The listing builds one solid part. Answer for the finished solid, in the listing's coordinates (mm). A direction names the side the tool comes from. Give positions to 0.01 mm unless a question says otherwise; leave off trailing zeros. Order: outer loops, then holes, each group sorted by start corner. A loop starts at its lowest first (then second) coordinate and runs counter-clockwise, first axis right, second up. Notation, with made-up numbers: (19.25, 87) - (63.25, 87) arc R15 cw to (63.25, 91) - close; hole circle Ø5 at (39.25, 38.5). An arc over 180 degrees is marked (long way). Answer as a JSON object with one key per item and string values. Group by question number.
Q1. Given pin 1 (3 mm diameter, centred on y = -23.5, z = 1.5, fed in from -X); pin 2 (5 mm diameter, centred on y = 24.5, z = -26, fed in from +X), each flat-ended and moving along its own axis, determine where each tip first touches the part or whether it passes through.
Q2. A cutting plane is placed at D-D, the plane z = -1. Give the vertices of the cut face in (x, y), and give its area (3 significant figures).
Q3. For faces 1 (the face through (0, 22, -26)), 2 (the face through (0, -29, 26)), 3 (the face through (6.35, 0, 1)), determine the directions among +Z, -Z, +X, -X, +Y, -Y from which every point of the face is accessible in a straight line to the end or side of a thin tool.
Q4. The mould has two halves that part along Z. Classify faces 4 (the face through (-3.219, -21.384, 27.96)), 5 (the face through (0, -31.75, 1)), 6 (the face through (0, 0, -38.1)): released by +Z, released by -Z, zero draft, split by the parting line, or undercut.
Q5. Consider line 1 (Y direction, x = 5.5, z = -22.5); line 2 (Y direction, x = -1.5, z = -2.5); line 3 (X direction, y = -26.5, z = 28.5). Determine where each line is inside the solid, lowest interval first.
Q6. A cutting plane is placed at A-A, the plane y = -25.4. Count the separate pieces of the cut face and the enclosed holes in it, and give its area (3 significant figures).
from build123d import *

# Parameters (mm, degrees)
BOSS_EXTRUDE1_DEPTH                           = 38.1
F_1_4_20_THREADED_C_BORE_D                    = 6.35
F_1_4_20_THREADED_C_BORE_CBORE_D              = 9.525
F_1_4_20_THREADED_C_BORE_CBORE_DEPTH          = 6.35
F_1_4_20_THREADED_C_BORE_OPPOSITE_D           = 6.35
F_1_4_20_THREADED_C_BORE_OPPOSITE_CBORE_D     = 9.525
F_1_4_20_THREADED_C_BORE_OPPOSITE_CBORE_DEPTH = 6.35


with BuildPart() as part:
    # Sketch2 → Boss-Extrude1 (new, symmetric)
    with BuildSketch(Plane.XY):
        Polygon((-6.35, 31.75), (6.35, 31.75), (6.35, -19.05), (6.35, -31.75), (-6.35, -31.75), (-6.35, 19.05), align=None)
    extrude(amount=BOSS_EXTRUDE1_DEPTH, both=True)

    # 1/4"-20 threaded c-bore (through all)
    with Locations(Plane.ZY.offset(6.35)):
        with Locations((-25.4, -25.4), (0, -25.4), (25.4, -25.4)):
            CounterBoreHole(F_1_4_20_THREADED_C_BORE_D / 2, F_1_4_20_THREADED_C_BORE_CBORE_D / 2, F_1_4_20_THREADED_C_BORE_CBORE_DEPTH)

    # 1/4"-20 threaded c-bore opposite (through all)
    with Locations(Plane(origin=(6.35, 0, 0), x_dir=(0, 0, -1), z_dir=(1, 0, 0))):
        with Locations((-25.4, 25.4), (0, 25.4), (25.4, 25.4)):
            CounterBoreHole(F_1_4_20_THREADED_C_BORE_OPPOSITE_D / 2, F_1_4_20_THREADED_C_BORE_OPPOSITE_CBORE_D / 2, F_1_4_20_THREADED_C_BORE_OPPOSITE_CBORE_DEPTH)


solid = part.part
Reply:
{
 "1": {"pin 1": "stops at x = 0", "pin 2": "stops at x = 0"},
 "2": {"outline": "(-6.35, -31.75) - (6.35, -31.75) - (6.35, -28.41) - (0, -28.41) - (0, -30.06) - (-6.35, -30.06) - close; (-6.35, -20.74) - (0, -20.74) - (0, -22.39) - (6.35, -22.39) - (6.35, 20.74) - (0, 20.74) - (0, 22.39) - (-6.35, 22.39) - close; (-6.35, 28.41) - (0, 28.41) - (0, 30.06) - (6.35, 30.06) - (6.35, 31.75) - (-6.35, 31.75) - close", "area": "612 mm^2"},
 "3": {"face 1": "+X", "face 2": "-X", "face 3": "+Z, -Z, +X, +Y, -Y"},
 "4": {"face 4": "undercut", "face 5": "zero draft", "face 6": "released by -Z"},
 "5": {"line 1": "y = -31.75 to -26.69, -24.11 to 21.62, 29.18 to 31.75", "line 2": "y = -31.75 to -29.45, -21.35 to 23.44, 27.36 to 31.75", "line 3": "x = 0 to 6.35"},
 "6": {"separate pieces": "4", "enclosed holes": "0", "area": "665 mm^2"}
}
